Input: part model. Units: mm. Frame: model coordinates. Face numbers are marked on the shaded views. A direction names the side the tool comes from. Round coordinates to 2 decimals unless told otherwise and drop trailing zeros. Order: outer loops, then holes, each group sorted by start corner. A loop starts at its lowest first (then second) coordinate and runs counter-clockwise, first axis right, second up. Notation, with made-up numbers: (-22, 39.5) -> (18, 39.5) arc R7 ccw to (18, 46.5) -> close; hole circle Ø7 at (1.25, -7). An arc over 180 degrees is marked (long way). Use a Markdown table: item, result.
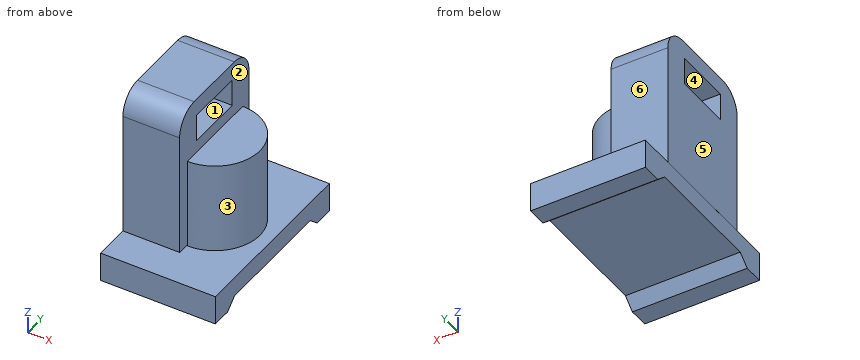
from build123d import *

# Parameters (mm, degrees)
SKETCH_W        = 39.101506
SKETCH_H        = 62.728786
PAD_DEPTH       = 10
POCKET_DEPTH    = 39.102506
SKETCH002_W     = 19.301168
SKETCH002_H     = 38.103164
PAD001_DEPTH    = 50
FILLET_R        = 8
PAD002_DEPTH    = 31
SKETCH004_W     = 19.757324
SKETCH004_H     = 9.317804
POCKET001_DEPTH = 19.302168


with BuildPart() as part:
    # Sketch → Pad (new body)
    with BuildSketch(Plane.XY):
        Rectangle(SKETCH_W, SKETCH_H)
    extrude(amount=PAD_DEPTH)

    # Sketch001 (on Face3 of Pad) → Pocket (cut, through all)
    with BuildSketch(Plane.YZ.offset(19.550753)):
        Polygon((-24.639747, 0), (-20.812978, 3.391465), (20.812978, 3.391465), (24.639747, 0), align=None)
    extrude(amount=-POCKET_DEPTH, mode=Mode.SUBTRACT)

    # Sketch002 (on Face8 of Pocket) → Pad001 (join)
    with BuildSketch(Plane.XY.offset(10)):
        with Locations((-9.90619, 0)):
            Rectangle(SKETCH002_W, SKETCH002_H)
    extrude(amount=PAD001_DEPTH)

    # Fillet
    fillet_edges = [part.edges().sort_by_distance(p)[0] for p in [
        (-9.90619, -19.051582, 60),
        (-9.90619, 19.051582, 60),
    ]]
    fillet(fillet_edges, radius=FILLET_R)

    # Sketch003 (on Face6 of Fillet) → Pad002 (join)
    with BuildSketch(Plane.XY.offset(10)):
        with BuildLine():
            ThreePointArc((0, -15.260272), (15.260272, 0), (0, 15.260272))
            Line((0, 0), (0, 15.260272))
            Line((0, 0), (0, -15.260272))
        make_face()
    extrude(amount=PAD002_DEPTH)

    # Sketch004 (on Face5 of Pad002) → Pocket001 (cut, through all)
    with BuildSketch(Plane.YZ.offset(-0.255606)):
        with Locations((0, 49.459888)):
            Rectangle(SKETCH004_W, SKETCH004_H)
    extrude(amount=-POCKET001_DEPTH, mode=Mode.SUBTRACT)


solid = part.part
1) Cut plane C-C on x = -8.5. Return loops of the section in (y, z).
Answer key:
| item | result |
|---|---|
| outline | (-31.36, 0) -> (-24.64, 0) -> (-20.81, 3.39) -> (20.81, 3.39) -> (24.64, 0) -> (31.36, 0) -> (31.36, 10) -> (19.05, 10) -> (19.05, 52) arc R8 ccw to (11.05, 60) -> (-11.05, 60) arc R8 ccw to (-19.05, 52) -> (-19.05, 10) -> (-31.36, 10) -> close; hole (-9.88, 44.8) -> (9.88, 44.8) -> (9.88, 54.12) -> (-9.88, 54.12) -> close |
2) Draft query along Y for the marked faces 4, 5 and 6. Return one class per face: released by +Y, released by -Y, zero draft, split by the parting line, or undercut.
Answer key:
| item | result |
|---|---|
| face 4 | undercut |
| face 5 | zero draft |
| face 6 | released by +Y |
3) Cut plane D-D on x = 9. Return loops of the section in (y, z), and give its area (3 significant figures).
Answer key:
| item | result |
|---|---|
| outline | (-31.36, 0) -> (-24.64, 0) -> (-20.81, 3.39) -> (20.81, 3.39) -> (24.64, 0) -> (31.36, 0) -> (31.36, 10) -> (12.32, 10) -> (12.32, 41) -> (-12.32, 41) -> (-12.32, 10) -> (-31.36, 10) -> close |
| area | 1,240 mm^2 |
4) Contact query for flat-ended pins moving along their axis: P1, Ø1, axis at x = 13, z = 23, coming from the -Y side; P2, Ø4.5, axis at x = 4.5, y = -6.5, coming from the +Z side; P3, Ø15.5, axis at x = -9, y = 0.5, coming from the -Z side; P4, Ø6, axis at y = 25, z = 38.5, coming from the -X side. Output: stop coordinate, or through.
Answer key:
| item | result |
|---|---|
| P1 | stops at y = -8.75 |
| P2 | stops at z = 41 |
| P3 | stops at z = 3.39 |
| P4 | passes through |
5) Set-up query: the marked faces 1, 2 and 3. Return all of +Z, -Z, +X, -X, +Y, -Y with unobstructed straight access to the full face (end or side cutting, diameter ignored); none if empty.
Answer key:
| item | result |
|---|---|
| face 1 | +X, -X |
| face 2 | +Z, +Y, -Y |
| face 3 | +Z, +X |
6) Ray query, probe 1 along Z at (x, y) = (-15.5, -3.5); probe 2 along Z at (x, y) = (10, 9); probe 3 along X at (y, z) = (-20, 5). Return the intervals inside material, ascending.
Answer key:
| item | result |
|---|---|
| probe 1 | z = 3.39 to 44.8, 54.12 to 60 |
| probe 2 | z = 3.39 to 41 |
| probe 3 | x = -19.55 to 19.55 |
7) Cut plane B-B on z = 19. Return loops of the section in (x, y), and give its area (3 significant figures).
Answer key:
| item | result |
|---|---|
| outline | (-19.56, -19.05) -> (-0.26, -19.05) -> (-0.26, 19.05) -> (-19.56, 19.05) -> close; (0, -15.26) arc R15.26 ccw to (0, 15.26) -> close |
| area | 1,100 mm^2 |
